Source: CAD feature listing. Evaluate the final solid. Frame: model axes, mm. A direction names the side the tool comes from. Give positions to 0.01 mm unless a question says otherwise; leave off trailing zeros. Order: outer loops, then holes, each group sorted by start corner. A loop starts at its lowest first (then second) coordinate and runs counter-clockwise, first axis right, second up. Notation, with made-up numbers: M 55,-29 L 103,-29 A22 cw 103,10 Z; hole C 39.25,37 d7. An arc over 180 degrees is marked long. One line per question, with ' | ' between items. Start each with the question number.
from build123d import *

# Parameters (mm, degrees)
SKETCH1_R           = 6
SKETCH1_R_2         = 2.625
BOSS_EXTRUDE1_DEPTH = 3
VARFILLET1_START    = 9
VARFILLET1_DEPTH    = 27
SKETCH3_R           = 0.75
CUT_EXTRUDE1_DEPTH  = 10


with BuildPart() as part:
    # Sketch1 → Boss-Extrude1 (new body)
    # profile 1 of 2: a face of its own
    with BuildSketch(Plane.XY):
        Circle(SKETCH1_R)
        Circle(SKETCH1_R_2, mode=Mode.SUBTRACT)
    # profile 2 of 2: a face of its own
    with BuildSketch(Plane.XY):
        with BuildLine():
            ThreePointArc((-6, 0), (0, 6), (6, 0))
            Line((6, 0), (6, 35))
            Line((6, 35), (-11.5, 35))
            Line((-11.5, 35), (-11.5, 10))
            Line((-11.5, 10), (-6, 10))
            Line((-6, 10), (-6, 0))
        make_face()
    extrude(amount=BOSS_EXTRUDE1_DEPTH)

    # VarFillet1: read off the stored shape, not the designer's step
    # VarFillet1 outline → VarFillet1 (cut)
    with BuildSketch(Plane(origin=(0, 0, 0), x_dir=(1, 0, 0), z_dir=(0, 1, 0)).offset(VARFILLET1_START)):
        with BuildLine():
            Line((-11.5, 0), (-11.5, -1))
            add(Edge.make_bspline(
                [(-11.5, -1), (-11.5, 0), (-10.5, 0)],
                knots=[0, 0, 0, 1, 1, 1], degree=2, weights=[1, 0.707106781, 1]))
            Line((-10.5, 0), (-11.5, 0))
        make_face()
        with BuildLine():
            add(Edge.make_bspline(
                [(-10.5, -3), (-11.5, -3), (-11.5, -2)],
                knots=[0, 0, 0, 1, 1, 1], degree=2, weights=[1, 0.707106781, 1]))
            Line((-11.5, -2), (-11.5, -3))
            Line((-11.5, -3), (-10.5, -3))
        make_face()
    extrude(amount=VARFILLET1_DEPTH, mode=Mode.SUBTRACT)

    # Sketch3 → Cut-Extrude1 (cut)
    with BuildSketch(Plane(origin=(0, 0, 0), x_dir=(-1, 0, 0), z_dir=(0, 0, -1))):
        with Locations((-1, 27.5)):
            Circle(SKETCH3_R)
    extrude(amount=-CUT_EXTRUDE1_DEPTH, mode=Mode.SUBTRACT)


solid = part.part
Item 1: Cut plane C-C on y = 1.5. Return the cut outline in (x, z), and give its area (3 significant figures).
Item 2: Cut plane D-D on z = 2.55. Count the separate pieces of the cut face and the enclosed holes in it, and give its area (3 significant figures).
Item 3: Mould query, pull axis Y, two halves, no side actions, for faces 1 (the flat face through (-3, 35, 1)), 2 (the flat face through (-2, 19, 3)), 3 (the cylindrical face through (2.5, 0.8, 1.5)), 4 (the cylindrical face through (0.285, 27.725, 1.479)). Classes: pulls with the +Y half, pulls with the -Y half, needs draft (parallel to the pull), parting line crosses it, or undercut.
Item 4: Cut plane A-A on x = 1. Return the cut outline in (y, z).
Item 5: Reachability of faces 5 (the flat face through (-6, 5, 1)), 6 (the cylindrical face through (0, -6, 1)) from +Z, -Z, +X, -X, +Y, -Y: full face, straight path, thin tool, end or side. Return the list, or none.
Item 6: Line query: line 1 (Y direction, x = 0, z = 1.4) (3 decimals); line 2 (Y direction, x = 1, z = 1.8); line 3 (X direction, y = 9, z = 0.25). Output: solid intervals per line, ascending.
Item 7: Pin query (flat end, axial travel): pin 1 Ø6 at (x, y) = (-4, 19) entering from -Z; pin 2 Ø0.9 at (x, z) = (-8.5, 2) entering from -Y. Return the tip coordinate at first contact, or that it passes through.
Item 8: Cut plane B-B on x = -1. Return the cut outline in (y, z).
Results are:
1) outline: M -6,0 L -2.15,0 L -2.15,3 L -6,3 Z; M 2.15,0 L 6,0 L 6,3 L 2.15,3 Z | area: 23.1 mm2
2) separate pieces: 1 | enclosed holes: 2 | area: 587 mm2
3) face 1: pulls with the +Y half | face 2: needs draft | face 3: undercut | face 4: undercut
4) outline: M -5.92,0 L -2.43,0 L -2.43,3 L -5.92,3 Z; M 2.43,0 L 26.75,0 L 26.75,3 L 2.43,3 Z; M 28.25,0 L 35,0 L 35,3 L 28.25,3 Z
5) face 5: +Z, -Z, -X, -Y | face 6: +Z, -Z, -Y
6) line 1: y = -6 to -2.625, 2.625 to 35 | line 2: y = -5.92 to -2.43, 2.43 to 26.75, 28.25 to 35 | line 3: x = -6 to 6
7) pin 1: stops at z = 0 | pin 2: stops at y = 10
8) outline: M -5.92,0 L -2.43,0 L -2.43,3 L -5.92,3 Z; M 2.43,0 L 35,0 L 35,3 L 2.43,3 Z
